```python
from build123d import *

# Parameters (mm, degrees)
BOSS_EXTRUDE1_DEPTH = 3


with BuildPart() as part:
    # Sketch1 → Boss-Extrude1 (new body)
    with BuildSketch(Plane.XY):
        Polygon((45.5, 78.667286245), (70.5, 53.667286245), (70.5, -46.332713755), (45.5, -71.332713755), (-54.5, -71.332713755), (-79.5, -46.332713755), (-79.5, 53.667286245), (-54.5, 78.667286245), align=None)
        Polygon((41.357864376, 68.667286245), (60.5, 49.525150622), (60.5, -42.190578131), (41.357864376, -61.332713755), (-50.357864376, -61.332713755), (-69.5, -42.190578131), (-69.5, 49.525150622), (-50.357864376, 68.667286245), align=None, mode=Mode.SUBTRACT)
    extrude(amount=BOSS_EXTRUDE1_DEPTH)


solid = part.part
```
Can you work these out from the model? Positions are in its coordinate system, mm. A direction names the side the tool comes from. Coordinates: 2 decimals unless noted, no trailing zeros. Write each loop counter-clockwise with the first axis right and the second up, starting at its lowest first coordinate (ties: lowest second). Pieces come first, ordered by that corner, then holes. Notation, with made-up numbers: M 41,86.25 L 74,86.25 A18 ccw 74,113.25 Z; hole C 68,49.5 d9. An arc over 180 degrees is marked long. Answer as CSV lines item,"result".
Item 1: We'd pull the mould along Y, two halves only. Please class faces 3 (the flat face through (-67.18, 65.99, 1.48)), 4 (the flat face through (58.175, -58.658, 1.479)), 5 (the flat face through (50.795, 59.23, 1.479)): +Y half, -Y half, draft (parallel to the pull), parting line (faces both ways), or undercut.
Geometry results:
face 3,"+Y half"
face 4,"-Y half"
face 5,"undercut"
Item 2: On a 3-axis mill with a long thin cutter (end or side, diameter ignored), from which of +Z, -Z, +X, -X, +Y, -Y can I reach the whole of each face in a straight line? I mean faces 1 (the flat face through (-60.063, 58.962, 1.479)), 2 (the flat face through (-66.82, -59.01, 1.48)). Say none if no direction works.
Geometry results:
face 1,"+Z, -Z"
face 2,"+Z, -Z, -X, -Y"
Item 3: Imagine slicing it at B-B on x = 39. List the corners of the cut face in (y, z) for me.
Geometry results:
outline,"M -71.33,0 L -61.33,0 L -61.33,3 L -71.33,3 Z; M 68.67,0 L 78.67,0 L 78.67,3 L 68.67,3 Z"
Item 4: Imagine slicing it at C-C on y = -34. List the corners of the cut face in (x, z) for me, plus the area to 3 significant figures.
Geometry results:
outline,"M -79.5,0 L -69.5,0 L -69.5,3 L -79.5,3 Z; M 60.5,0 L 70.5,0 L 70.5,3 L 60.5,3 Z"
area,"60.0 mm2"
Item 5: Please list where these lines run through material, in increasing order: line 1 along X through (y, z) = (32, 1.45); line 2 along Y through (x, z) = (19, 2.4); line 3 along X through (y, z) = (51, 2).
Geometry results:
line 1,"x = -79.5 to -69.5, 60.5 to 70.5"
line 2,"y = -71.33 to -61.33, 68.67 to 78.67"
line 3,"x = -79.5 to -68.03, 59.03 to 70.5"
Item 6: Imagine slicing it at A-A on z = 1.15. List the corners of the cut face in (x, y) for me.
Geometry results:
outline,"M -79.5,-46.33 L -54.5,-71.33 L 45.5,-71.33 L 70.5,-46.33 L 70.5,53.67 L 45.5,78.67 L -54.5,78.67 L -79.5,53.67 Z; hole M -69.5,-42.19 L -50.36,-61.33 L 41.36,-61.33 L 60.5,-42.19 L 60.5,49.53 L 41.36,68.67 L -50.36,68.67 L -69.5,49.53 Z"
